```python
from build123d import *

# Parameters (mm, degrees)
F0_R     = 1.25
F1_DEPTH = 59
F2_W     = 10
F2_H     = 7.0094654113
F2_H_2   = 7.1141358241
F3_DEPTH = 12.0799340399
F5_D     = 2.2606


with BuildPart() as f1:
    # F0 (on Front) → F1 (new body)
    with BuildSketch(Plane.XZ):
        with BuildLine():
            Line((0, 0.9144042292), (0, 0))
            Line((0, 0), (11, 0))
            Line((11, 0), (11, 1))
            Line((11, 1), (1.0663817193, 1))
            ThreePointArc((1.0663817193, 1), (0.5410811762, 0.8589018219), (0, 0.9144042292))
        make_face()
        with BuildLine():
            Line((0, 1), (0, 0.9144042292))
            ThreePointArc((0, 0.9144042292), (0.5410811762, 0.8589018219), (1.0663817193, 1))
            Line((1.0663817193, 1), (0, 1))
        make_face()
        with BuildLine():
            ThreePointArc((1.9210659601, 2.354092896), (-0.4784897802, 3.5544259623), (0, 0.9144042292))
            Line((0, 0.9144042292), (0, 1))
            Line((0, 1), (1.0663817193, 1))
            ThreePointArc((1.0663817193, 1), (1.6895244022, 1.5534599085), (1.9210659601, 2.354092896))
        make_face()
        with Locations((0.4210659601, 2.354092896)):
            Circle(F0_R, mode=Mode.SUBTRACT)
    extrude(amount=F1_DEPTH)

    # F2 (on face) → F3 (cut, through all)
    with BuildSketch(Plane.YZ.offset(11)):
        with Locations((-45, 4.5047327057)):
            Rectangle(F2_W, F2_H)
        with Locations((-25, 4.5570679121)):
            Rectangle(F2_W, F2_H_2)
        with Locations((-5, 4.5570679121)):
            Rectangle(F2_W, F2_H_2)
    extrude(amount=-F3_DEPTH, mode=Mode.SUBTRACT)

    # F5 (through all)
    with Locations(Plane.XY.offset(1)):
        with Locations((5.463800393, -6.5), (5.463800393, -29.5), (5.463800393, -52.5)):
            Hole(F5_D / 2)


solid = f1.part
```
Model file for the job. Use its own axes, mm. A direction names the side the tool comes from. Give positions to 0.01 mm unless a question says otherwise; leave off trailing zeros. Loops run counter-clockwise (first coordinate to the right, second up) from the corner with the lowest first, then second, coordinate; pieces in that order, holes last. Notation, with made-up numbers: (77, -3.5) -> (84, -3.5) arc R21 ccw to (84, 34.5) -> close; hole circle Ø11 at (8, 24.5). An arc over 180 degrees is marked (long way). Use CSV: the item, a comma, the result in double quotes. Start each with the question number.
1) Tool access for faces 4 (the flat face through (0, -29.1, 0.5)), 5 (the cylindrical face through (4.94, -7.5, 0.49)): list every direction of +Z, -Z, +X, -X, +Y, -Y with a clear straight run to the whole face (end or side of a thin tool).
2) Flat gauge pins, fed straight in: pin 1 Ø2 at (x, y) = (1.5, -20.5) entering from +Z; pin 2 Ø2.5 at (x, y) = (5.46, -6.5) entering from +Z; pin 3 Ø3 at (x, y) = (2.5, -8) entering from -Z. Where does each tip first touch, or does it go through?
3) Slice it at C-C on x = 0.5. Give the cut face in (y, z).
4) Wall check: line 1 (Y direction, x = 6.25, z = 0.5); line 2 (Z direction, x = 0.5, y = -39); line 3 (Z direction, x = 7.5, y = -19). Give the ranges that are in metal, low to high.
5) Mould opens along Z. For faces 1 (the cylindrical face through (4.856, -28.547, 0.493)), 2 (the cylindrical face through (0.15, -14.93, 1.134)), 3 (the flat face through (7, -29, 0)) say: released by +Z, released by -Z, zero draft, split by the parting line, or undercut.
6) Slice it at D-D on y = -29.5. Give the cut face in (x, z), plus the area to 3 significant figures.
7) Slice it at A-A on y = -52.5. Give the cut face in (x, z), plus the area to 3 significant figures.
8) Slice it at B-B on y = -14.5. Give the cut face in (x, z), plus the area to 3 significant figures.
Computed values:
1,face 4,"-Z, -X, +Y, -Y"
1,face 5,"+Z, -Z"
2,pin 1,"stops at z = 3.84"
2,pin 2,"stops at z = 1"
2,pin 3,"stops at z = 0"
3,outline,"(-59, 0) -> (0, 0) -> (0, 1) -> (-10, 1) -> (-10, 1.11) -> (-20, 1.11) -> (-20, 1) -> (-30, 1) -> (-30, 1.11) -> (-40, 1.11) -> (-40, 1) -> (-50, 1) -> (-50, 1.11) -> (-59, 1.11) -> close; (-59, 3.6) -> (-50, 3.6) -> (-50, 3.85) -> (-59, 3.85) -> close; (-40, 3.6) -> (-30, 3.6) -> (-30, 3.85) -> (-40, 3.85) -> close; (-20, 3.6) -> (-10, 3.6) -> (-10, 3.85) -> (-20, 3.85) -> close"
4,line 1,"y = -59 to -53.31, -51.69 to -30.31, -28.69 to -7.31, -5.69 to 0"
4,line 2,"z = 0 to 1.11, 3.6 to 3.85"
4,line 3,"z = 0 to 1"
5,face 1,"zero draft"
5,face 2,"undercut"
5,face 3,"released by -Z"
6,outline,"(-0.22, 1) arc R1.5 ccw to (0, 0.91) -> (0, 0) -> (4.33, 0) -> (4.33, 1) -> close; (6.59, 0) -> (11, 0) -> (11, 1) -> (6.59, 1) -> close"
6,area,"8.75 mm^2"
7,outline,"(0, 0) -> (4.33, 0) -> (4.33, 1) -> (1.07, 1) arc R1.5 ccw (long way) to (0, 0.91) -> close; (6.59, 0) -> (11, 0) -> (11, 1) -> (6.59, 1) -> close; hole circle Ø2.5 at (0.42, 2.35)"
7,area,"10.8 mm^2"
8,outline,"(0, 0) -> (11, 0) -> (11, 1) -> (1.07, 1) arc R1.5 ccw (long way) to (0, 0.91) -> close; hole circle Ø2.5 at (0.42, 2.35)"
8,area,"13.0 mm^2"
